Build history of the part. All positions in model axes, mm. A direction names the side the tool comes from. Round coordinates to 2 decimals unless told otherwise and drop trailing zeros. Order: outer loops, then holes, each group sorted by start corner. A loop starts at its lowest first (then second) coordinate and runs counter-clockwise, first axis right, second up. Notation, with made-up numbers: (15, -22) -> (66, -22) arc R30 cw to (66, 11) -> close; hole circle Ø10 at (25, 84). An arc over 180 degrees is marked (long way). Answer as a JSON object with one key per item and string values.
from build123d import *

# Parameters (mm, degrees)
SK_BASE_W             = 50
SK_BASE_H             = 50
EX_BASE_DEPTH         = 4
SK_DECKHOLES_R        = 2.15
CUT_DECKHOLES_DEPTH   = 4
SK_COLUMN_W           = 30
SK_COLUMN_H           = 30
EX_COLUMN_DEPTH       = 44.8
SK_TOP_W              = 58
SK_TOP_H              = 58
EX_TOP_DEPTH          = 4
SK_INSERTS_M25_R      = 1.8
CUT_INSERTS_M25_DEPTH = 4


with BuildPart() as part:
    # SK_Base → EX_Base (new body)
    with BuildSketch(Plane(origin=(0, 0, 0), x_dir=(1, 0, 0), z_dir=(0, 1, 0))):
        Rectangle(SK_BASE_W, SK_BASE_H)
    extrude(amount=EX_BASE_DEPTH)

    # SK_DeckHoles → CUT_DeckHoles (cut)
    with BuildSketch(Plane(origin=(0, 0, 0), x_dir=(1, 0, 0), z_dir=(0, 1, 0))):
        with Locations(Location((20, -20, 0), (0, 0, 270))):
            Circle(SK_DECKHOLES_R)
        with Locations(Location((-20, -20, 0), (0, 0, 270))):
            Circle(SK_DECKHOLES_R)
        with Locations(Location((20, 20, 0), (0, 0, 270))):
            Circle(SK_DECKHOLES_R)
        with Locations(Location((-20, 20, 0), (0, 0, 270))):
            Circle(SK_DECKHOLES_R)
    extrude(amount=CUT_DECKHOLES_DEPTH, mode=Mode.SUBTRACT)

    # SK_Column → EX_Column (add)
    with BuildSketch(Plane(origin=(0, 4, 0), x_dir=(1, 0, 0), z_dir=(0, 1, 0))):
        Rectangle(SK_COLUMN_W, SK_COLUMN_H)
    extrude(amount=EX_COLUMN_DEPTH)

    # SK_Top → EX_Top (add)
    with BuildSketch(Plane(origin=(0, 48.8, 0), x_dir=(1, 0, 0), z_dir=(0, 1, 0))):
        Rectangle(SK_TOP_W, SK_TOP_H)
    extrude(amount=EX_TOP_DEPTH)

    # SK_Inserts_M25 → CUT_Inserts_M25 (cut)
    with BuildSketch(Plane(origin=(0, 52.8, 0), x_dir=(1, 0, 0), z_dir=(0, 1, 0))):
        with Locations(Location((23.4, -4.93, 0), (0, 0, 270))):
            Circle(SK_INSERTS_M25_R)
        with Locations(Location((-23.4, -4.93, 0), (0, 0, 270))):
            Circle(SK_INSERTS_M25_R)
        with Locations(Location((0, 23.39, 0), (0, 0, 270))):
            Circle(SK_INSERTS_M25_R)
    extrude(amount=-CUT_INSERTS_M25_DEPTH, mode=Mode.SUBTRACT)


solid = part.part
1) Cut at A-A, the plane x = -20. Give the cut face in (y, z), plus the area to 3 significant figures.
Checked values:
{"outline": "(0, -25) -> (4, -25) -> (4, -22.15) -> (0, -22.15) -> close; (0, -17.85) -> (4, -17.85) -> (4, 17.85) -> (0, 17.85) -> close; (0, 22.15) -> (4, 22.15) -> (4, 25) -> (0, 25) -> close; (48.8, -29) -> (52.8, -29) -> (52.8, 29) -> (48.8, 29) -> close", "area": "398 mm²"}
2) Probe L1, parallel to X at y = 1.8, z = -20; L2, parallel to Y at x = 8, z = -19; L3, parallel to X at y = 50.6, z = 4.93. List the from-to ranges inside material, lowest first. Write a range as from..to.
Checked values:
{"L1": "x = -25..-22.15, -17.85..17.85, 22.15..25", "L2": "y = 0..4, 48.8..52.8", "L3": "x = -29..-25.2, -21.6..21.6, 25.2..29"}
3) Cut at B-B, the plane z = 20. Give the cut face in (x, y), plus the area to 3 significant figures.
Checked values:
{"outline": "(-29, 48.8) -> (29, 48.8) -> (29, 52.8) -> (-29, 52.8) -> close; (-25, 0) -> (-22.15, 0) -> (-22.15, 4) -> (-25, 4) -> close; (-17.85, 0) -> (17.85, 0) -> (17.85, 4) -> (-17.85, 4) -> close; (22.15, 0) -> (25, 0) -> (25, 4) -> (22.15, 4) -> close", "area": "398 mm²"}
4) Pull direction X, two halves, no side cores. Call faces 5 (the face through (17.9, 1.97, -20.47)), 6 (the face through (-25, 2, 0)), 7 (the face through (0, 26, 15)): pulls with the +X half, pulls with the -X half, needs draft (parallel to the pull), parting line crosses it, or undercut.
Checked values:
{"face 5": "undercut", "face 6": "pulls with the -X half", "face 7": "needs draft"}
5) Which spindle directions (+Z, -Z, +X, -X, +Y, -Y) get a long thin tool onto all of the face, cutting with end or side? Do faces 1 (the face through (21.643, 50.828, 4.54)), 2 (the face through (-17, 4, 0)), 3 (the face through (0, 26, -15)), 4 (the face through (25, 2, 0)). Say none if no direction does.
Checked values:
{"face 1": "+Y", "face 2": "none", "face 3": "-Z, +X, -X", "face 4": "+Z, -Z, +X, -Y"}
6) Cut at C-C, the plane x = 0. Give the cut face in (y, z), plus the area to 3 significant figures.
Checked values:
{"outline": "(0, -25) -> (4, -25) -> (4, -15) -> (48.8, -15) -> (48.8, -21.59) -> (52.8, -21.59) -> (52.8, 29) -> (48.8, 29) -> (48.8, 15) -> (4, 15) -> (4, 25) -> (0, 25) -> close; (48.8, -29) -> (52.8, -29) -> (52.8, -25.19) -> (48.8, -25.19) -> close", "area": "1,760 mm²"}
7) Flat gauge pins, fed straight in: pin 1 Ø24 at (y, z) = (36.5, 3.5) entering from -X; pin 2 Ø12 at (y, z) = (44, -20) entering from -X; pin 3 Ø1.2 at (y, z) = (2, 6) entering from -X; pin 4 Ø1.2 at (x, y) = (4, 2.5) entering from -Z. Where does each tip first touch, or does it go through?
Checked values:
{"pin 1": "stops at x = -15", "pin 2": "stops at x = -29", "pin 3": "stops at x = -25", "pin 4": "stops at z = -25"}
8) Cut at D-D, the plane z = 5.5. Give the cut face in (x, y), plus the area to 3 significant figures.
Checked values:
{"outline": "(-29, 48.8) -> (-25.11, 48.8) -> (-25.11, 52.8) -> (-29, 52.8) -> close; (-25, 0) -> (25, 0) -> (25, 4) -> (15, 4) -> (15, 48.8) -> (21.69, 48.8) -> (21.69, 52.8) -> (-21.69, 52.8) -> (-21.69, 48.8) -> (-15, 48.8) -> (-15, 4) -> (-25, 4) -> close; (25.11, 48.8) -> (29, 48.8) -> (29, 52.8) -> (25.11, 52.8) -> close", "area": "1,750 mm²"}
